from build123d import *

# Parameters (mm, degrees)
F0_W     = 1.25
F0_H     = 9
F3_COUNT = 6
F5_SIZE  = 0.2
F6_SIZE  = 0.2


with BuildPart() as f1:
    # F0 (on Top) → F1 (revolve)
    with BuildSketch(Plane.XY):
        Polygon((2.5, -7.5), (0, -7.5), (-2.5, -7.5), (-2.5, -11.5), (-1.25, -11.5), (-1.25, -9.5), (0, -9.5), (1.25, -9.5), (1.25, -11.5), (2.5, -11.5), align=None)
    revolve(axis=Axis((6.057695, 0, 0), (1, 0, 0)))


with BuildPart() as f2:
    # F0 (on Top) → F2 (revolve)
    with BuildSketch(Plane.XY):
        with Locations((0.625, 8.5)):
            Rectangle(F0_W, F0_H)
    revolve(axis=Axis((0, 8.5, 0), (0, -1, 0)))


with BuildPart() as f3_1:
    # F3: instance of F2
    add(f2.part.rotate(Axis((6.057695, 0, 0), (1, 0, 0)), 1 * 360 / F3_COUNT))


with BuildPart() as f3_2:
    # F3: instance of F2
    add(f2.part.rotate(Axis((6.057695, 0, 0), (1, 0, 0)), 2 * 360 / F3_COUNT))


with BuildPart() as f3_3:
    # F3: instance of F2
    add(f2.part.rotate(Axis((6.057695, 0, 0), (1, 0, 0)), 3 * 360 / F3_COUNT))


with BuildPart() as f3_4:
    # F3: instance of F2
    add(f2.part.rotate(Axis((6.057695, 0, 0), (1, 0, 0)), 4 * 360 / F3_COUNT))


with BuildPart() as f3_5:
    # F3: instance of F2
    add(f2.part.rotate(Axis((6.057695, 0, 0), (1, 0, 0)), 5 * 360 / F3_COUNT))


with BuildPart() as f1_1:
    add(f1.part)

    # F4: cut F2, F3_2, F3_1, F3_3, F3_4, F3_5
    add(f2.part, mode=Mode.SUBTRACT)
    add(f3_2.part, mode=Mode.SUBTRACT)
    add(f3_1.part, mode=Mode.SUBTRACT)
    add(f3_3.part, mode=Mode.SUBTRACT)
    add(f3_4.part, mode=Mode.SUBTRACT)
    add(f3_5.part, mode=Mode.SUBTRACT)

    # F5
    f5_edges = [f1_1.edges().sort_by_distance(p)[0] for p in [
        (2.5, 11.5, 0),
        (-2.5, 11.5, 0),
    ]]
    chamfer(f5_edges, length=F5_SIZE)

    # F6
    f6_edges = [f1_1.edges().sort_by_distance(p)[0] for p in [
        (-1.25, 11.5, 0),
        (1.25, 11.5, 0),
        (2.5, 7.5, 0),
        (-2.5, 7.5, 0),
    ]]
    chamfer(f6_edges, length=F6_SIZE)


solid = f1_1.part
The model under review builds one solid part; all positions refer to its coordinate system, in mm. A direction names the side the tool comes from. Give positions to 0.01 mm unless a question says otherwise; leave off trailing zeros. Write each loop counter-clockwise with the first axis right and the second up, starting at its lowest first coordinate (ties: lowest second). Pieces come first, ordered by that corner, then holes. Notation, with made-up numbers: M 55.5,74 L 79.5,74 A20 ccw 79.5,98 Z; hole C 83.5,72 d2. An arc over 180 degrees is marked long. One line per question, with ' | ' between items. Start each with the question number.
Item 1: We need section C-C on x = -1.9. Write out the cut boundary in (y, z).
Item 2: Draft analysis for pull direction X (two halves, no side actions). For faces 4 (the cylindrical face through (-1.9, 1.5, -11.4)), 5 (the cylindrical face through (0, -0.1, -9.5)), 6 (the flat face through (2.5, -7.4, -2.7)), state which applies: released by +X, released by -X, zero draft, split by the parting line, or undercut.
Item 3: We need section B-B on x = 0. Write out the cut boundary in (y, z), plus the area to 3 significant figures.
Item 4: We need section A-A on y = 0. Write out the cut boundary in (x, z).
Item 5: Wall thickness on line 1 (X direction, y = 10.5, z = 4); line 2 (Z direction, x = 0.45, y = 0); line 3 (Y direction, x = -0.15, z = 5.5): over which ranges is each line inside the solid? List them lowest first. Write a range as from..to.
Item 6: For pin 1 (12 mm diameter, centred on y = 2, z = -1.5, fed in from -X); pin 2 (9 mm diameter, centred on y = 0, z = 0, fed in from -X); pin 3 (1 mm diameter, centred on x = -1, y = -5.5, fed in from +Z); pin 4 (1.5 mm diameter, centred on x = -1.5, z = -1.5, fed in from +Y), all flat-tipped, find the tip position at first contact; note any pin that passes through.
Item 7: For faces 1 (the flat face through (-1.25, 2.6, -9.3)), 2 (the cylindrical face through (0, 8.2, -4.8)), 3 (the cylindrical face through (0.02, -8.26, -4.69)), list the 3-axis set-ups (+Z, -Z, +X, -X, +Y, -Y) from which the entire face can be reached by the end or side of a thin tool; tool diameter is ignored.
Results found:
1) outline: C 0,0 d23; hole C 0,0 d15
2) face 4: zero draft | face 5: undercut | face 6: released by +X
3) outline: M -9.42,-1.25 A9.5 ccw -5.79,-7.53 L -4.78,-5.78 A7.5 cw -7.4,-1.25 Z; M -9.42,1.25 L -7.4,1.25 A7.5 cw -4.78,5.78 L -5.79,7.53 A9.5 ccw Z; M -3.63,-8.78 A9.5 ccw 3.63,-8.78 L 2.62,-7.03 A7.5 cw -2.62,-7.03 Z; M -3.63,8.78 L -2.62,7.03 A7.5 cw 2.62,7.03 L 3.63,8.78 A9.5 ccw Z; M 4.78,-5.78 L 5.79,-7.53 A9.5 ccw 9.42,-1.25 L 7.4,-1.25 A7.5 cw Z; M 4.78,5.78 A7.5 cw 7.4,1.25 L 9.42,1.25 A9.5 ccw 5.79,7.53 Z | area: 76.7 mm2
4) outline: M -2.5,-11.3 L -2.3,-11.5 L -1.45,-11.5 L -1.25,-11.3 L -1.25,-9.5 L 1.25,-9.5 L 1.25,-11.3 L 1.45,-11.5 L 2.3,-11.5 L 2.5,-11.3 L 2.5,-7.7 L 2.3,-7.5 L -2.3,-7.5 L -2.5,-7.7 Z; M -2.5,7.7 L -2.3,7.5 L 2.3,7.5 L 2.5,7.7 L 2.5,11.3 L 2.3,11.5 L 1.45,11.5 L 1.25,11.3 L 1.25,9.5 L -1.25,9.5 L -1.25,11.3 L -1.45,11.5 L -2.3,11.5 L -2.5,11.3 Z
5) line 1: x = -2.5..-1.25, 1.25..2.5 | line 2: z = -9.5..-7.5, 7.5..9.5 | line 3: y = -7.75..-5.1, 5.1..7.75
6) pin 1: stops at x = -2.5 | pin 2: passes through | pin 3: stops at z = 10.22 | pin 4: stops at y = 11.48
7) face 1: none | face 2: -Z, +Y | face 3: -Z, -Y
